Verification items for the finished model (mm, model axes). A direction names the side the tool comes from. Give positions to 0.01 mm unless a question says otherwise; leave off trailing zeros. Order: outer loops, then holes, each group sorted by start corner. A loop starts at its lowest first (then second) coordinate and runs counter-clockwise, first axis right, second up. Notation, with made-up numbers: (64, -23) - (111, -23) arc R20 ccw to (111, -7) - close; hole circle Ø9 at (80, 43.5). An arc over 180 degrees is marked (long way). Answer as a JSON object with one key per item and string values.
```python
from build123d import *

# Parameters (mm, degrees)
BOSS_EXTRUDE1_DEPTH             = 60
BOSS_EXTRUDE1_DRAFT             = -2
CBORE_FOR_M5_SBHCS1_D           = 5.8
CBORE_FOR_M5_SBHCS1_CBORE_D     = 11.5
CBORE_FOR_M5_SBHCS1_CBORE_DEPTH = 55


with BuildPart() as part:
    # Sketch1 → Boss-Extrude1 (with draft: the straight prism first)
    with BuildSketch(Plane(origin=(0, 0, 0), x_dir=(1, 0, 0), z_dir=(0, 1, 0))):
        Polygon((0, 0), (40, 0), (40, 20), (20, 20), (20, 45), (0, 45), align=None)
    extrude(amount=-BOSS_EXTRUDE1_DEPTH)
    # Boss-Extrude1: the draft: its side faces are tilted about the plane it starts from
    boss_extrude1_sides = [part.faces().sort_by_distance(p)[0] for p in [
        (20, -30, 0),
        (40, -30, -10),
        (30, -30, -20),
        (20, -30, -32.5),
        (10, -30, -45),
        (0, -30, -22.5),
    ]]
    draft(boss_extrude1_sides, Plane(origin=(0, 0, 0), x_dir=(1, 0, 0), z_dir=(0, 1, 0)), BOSS_EXTRUDE1_DRAFT)

    # CBORE for M5 SBHCS1 (through all)
    with Locations(Plane(origin=(0, -60, 0), x_dir=(-1, 0, 0), z_dir=(0, -1, 0))):
        with Locations((-10, 10), (-30, 10), (-10, 35)):
            CounterBoreHole(CBORE_FOR_M5_SBHCS1_D / 2, CBORE_FOR_M5_SBHCS1_CBORE_D / 2, CBORE_FOR_M5_SBHCS1_CBORE_DEPTH)


solid = part.part
```
(1) Access from +Z, -Z, +X, -X, +Y, -Y to the whole of each face (thin tool, end or side, straight path). Record for faces 1 (the cylindrical face through (4.516, -32.885, -11.727)), 2 (the cylindrical face through (7.1, -2.5, -10.1)).
Computed values:
{"face 1": "-Y", "face 2": "+Y, -Y"}
(2) Section check B-B (x = 10). Record the cut outline in (y, z).
Computed values:
{"outline": "(-60, -42.9) - (0, -45) - (0, -37.9) - (-5, -37.9) - (-5, -40.75) - (-60, -40.75) - close; (-60, -29.25) - (-5, -29.25) - (-5, -32.1) - (0, -32.1) - (0, -12.9) - (-5, -12.9) - (-5, -15.75) - (-60, -15.75) - close; (-60, -4.25) - (-5, -4.25) - (-5, -7.1) - (0, -7.1) - (0, 0) - (-60, -2.1) - close"}
(3) Section check A-A (z = -35). Record the cut outline in (x, y).
Computed values:
{"outline": "(0, 0) - (2.1, -60) - (4.25, -60) - (4.25, -5) - (7.1, -5) - (7.1, 0) - close; (12.9, -5) - (15.75, -5) - (15.75, -60) - (17.9, -60) - (20, 0) - (12.9, 0) - close"}
(4) Section check C-C (z = -10). Record the cut outline in (x, y).
Computed values:
{"outline": "(0, 0) - (2.1, -60) - (4.25, -60) - (4.25, -5) - (7.1, -5) - (7.1, 0) - close; (12.9, -5) - (15.75, -5) - (15.75, -60) - (24.25, -60) - (24.25, -5) - (27.1, -5) - (27.1, 0) - (12.9, 0) - close; (32.9, -5) - (35.75, -5) - (35.75, -60) - (37.9, -60) - (40, 0) - (32.9, 0) - close"}
(5) Release check for a two-part mould opening along Z. For faces 3 (the flat face through (12, -60, -18)), 4 (the cylindrical face through (32.766, -2.465, -10.871)), 5 (the cylindrical face through (7.699, -2.465, -33.235)) record: pulls with the +Z half, pulls with the -Z half, needs draft (parallel to the pull), parting line crosses it, or undercut.
Computed values:
{"face 3": "needs draft", "face 4": "undercut", "face 5": "undercut"}
(6) Material ranges on line 1 along X through (y, z) = (-1, -10); line 2 along Z through (x, y) = (10, -43); line 3 along Z through (x, y) = (7.5, -14.5), recorded low to high. Write a range as [from, to].
Computed values:
{"line 1": "x = [0.03, 7.1], [12.9, 27.1], [32.9, 39.97]", "line 2": "z = [-43.5, -40.75], [-29.25, -15.75], [-4.25, -1.5]", "line 3": "z = [-44.49, -40.18], [-29.82, -15.18], [-4.82, -0.51]"}
(7) Section check D-D (y = -24). Record the cut outline in (x, z), then the cut area to 3 significant figures.
Computed values:
{"outline": "(0.84, -44.16) - (19.16, -44.16) - (19.16, -19.16) - (39.16, -19.16) - (39.16, -0.84) - (0.84, -0.84) - close; hole circle Ø11.5 at (10, -35); hole circle Ø11.5 at (10, -10); hole circle Ø11.5 at (30, -10)", "area": "849 mm²"}
(8) Gauge pin test, flat ends, axial feed: pin 1 Ø5 at (x, z) = (10, -35) entering from +Y; pin 2 Ø2 at (x, y) = (14.5, -18) entering from +Z; pin 3 Ø8 at (y, z) = (-27, -17.5) entering from -X; pin 4 Ø2 at (y, z) = (-48, -31) entering from +X. Record the tip position at first contact, or that the pin passes through.
Computed values:
{"pin 1": "passes through", "pin 2": "stops at z = -0.59", "pin 3": "stops at x = 0.8", "pin 4": "stops at x = 18.36"}
